```python
from build123d import *

# Parameters (mm, degrees)
TABAN_FLAN_1_DEPTH    = 10
IZIM2_R               = 25
IZIM2_R_2             = 4.25
IZIM2_R_3             = 5.5
IZIM2_R_4             = 3.25
KES_EKSTR_ZYON1_DEPTH = 10
RADYUS2_R             = 50
RADYUS3_R             = 30
RADYUS4_R             = 10
RADYUS5_R             = 50
RADYUS6_R             = 10
RADYUS7_R             = 5
IZIM3_R               = 2.5
KES_EKSTR_ZYON2_DEPTH = 29


# Sheet-metal steps are written as plain solids
with BuildPart() as part:
    # Çizim1 → Taban-Flanş1 (new body)
    with BuildSketch(Plane.XY):
        Polygon((0, 120), (-400, 120), (-400, 20), (-420, 20), (-420, -55), (-360, -55), (-330, -40), (-250, -40), (-200, -30), (-135, -30), (-135, -90), (-100, -90), (-100, -30), (0, -30), (0, 0), align=None)
    extrude(amount=-TABAN_FLAN_1_DEPTH)

    # Çizim2 → Kes-Ekstrüzyon1 (cut)
    with BuildSketch(Plane.XY):
        with Locations((-310, 45)):
            Circle(IZIM2_R)
        with Locations((-351.5, 86.5)):
            Circle(IZIM2_R_2)
        with Locations((-268.5, 86.5)):
            Circle(IZIM2_R_2)
        with Locations((-351.5, 3.5)):
            Circle(IZIM2_R_2)
        with Locations((-268.5, 3.5)):
            Circle(IZIM2_R_2)
        with Locations((-60, 55)):
            Circle(IZIM2_R_3)
        with Locations((-160, 55)):
            Circle(IZIM2_R_3)
        with Locations((-160, 15)):
            Circle(IZIM2_R_3)
        with Locations((-60, 15)):
            Circle(IZIM2_R_3)
        with Locations((-117.5, -75)):
            Circle(IZIM2_R_3)
        with Locations((-405, 10)):
            Circle(IZIM2_R_4)
        with Locations((-405, -40)):
            Circle(IZIM2_R_4)
    extrude(amount=-KES_EKSTR_ZYON1_DEPTH, mode=Mode.SUBTRACT)

    # Radyus2
    radyus2_edges = [part.edges().sort_by_distance(p)[0] for p in [
        (-400, 120, -5),
    ]]
    fillet(radyus2_edges, radius=RADYUS2_R)

    # Radyus3
    radyus3_edges = [part.edges().sort_by_distance(p)[0] for p in [
        (0, 120, -5),
    ]]
    fillet(radyus3_edges, radius=RADYUS3_R)

    # Radyus4
    radyus4_edges = [part.edges().sort_by_distance(p)[0] for p in [
        (0, -30, -5),
        (-100, -30, -5),
        (-100, -90, -5),
        (-135, -90, -5),
        (-135, -30, -5),
    ]]
    fillet(radyus4_edges, radius=RADYUS4_R)

    # Radyus5
    radyus5_edges = [part.edges().sort_by_distance(p)[0] for p in [
        (-200, -30, -5),
        (-250, -40, -5),
        (-330, -40, -5),
        (-360, -55, -5),
    ]]
    fillet(radyus5_edges, radius=RADYUS5_R)

    # Radyus6
    radyus6_edges = [part.edges().sort_by_distance(p)[0] for p in [
        (-420, -55, -5),
        (-420, 20, -5),
    ]]
    fillet(radyus6_edges, radius=RADYUS6_R)

    # Radyus7
    radyus7_edges = [part.edges().sort_by_distance(p)[0] for p in [
        (-400, 20, -5),
    ]]
    fillet(radyus7_edges, radius=RADYUS7_R)

    # Çizim3 → Kes-Ekstrüzyon2 (cut)
    with BuildSketch(Plane(origin=(0, 0, -10), x_dir=(-1, 0, 0), z_dir=(0, 0, -1))):
        with Locations((232.5, 72.5)):
            Circle(IZIM3_R)
        with Locations((232.5, 17.5)):
            Circle(IZIM3_R)
        with Locations((387.5, 17.5)):
            Circle(IZIM3_R)
        with Locations((387.5, 72.5)):
            Circle(IZIM3_R)
    extrude(amount=-KES_EKSTR_ZYON2_DEPTH, mode=Mode.SUBTRACT)


solid = part.part
```
Model file for the job. Use its own axes, mm. A direction names the side the tool comes from. Coordinates: 2 decimals unless noted, no trailing zeros. Order: outer loops, then holes, each group sorted by start corner. A loop starts at its lowest first (then second) coordinate and runs counter-clockwise, first axis right, second up. Notation, with made-up numbers: (-0.75, 14) - (46.25, 14) arc R18 cw to (46.25, 23) - close; hole circle Ø7 at (-19, 20.5). An arc over 180 degrees is marked (long way). Return JSON: item names as keys, results as strings. Group by question number.
1) Mould opens along Y. For faces 1 (the flat face through (-213, 40, -10)), 2 (the cylindrical face through (-65.495, 15.242, -4.93)), 3 (the flat face through (-345.06, -47.53, -4.93)) say: released by +Y, released by -Y, zero draft, split by the parting line, or undercut.
2) Tool access for faces 4 (the cylindrical face through (-360.47, -53.7, -5.07)), 5 (the flat face through (-51, -30, -5)), 6 (the cylindrical face through (-65.495, 55.242, -4.93)), 7 (the flat face through (-400, 48, -5)), 8 (the flat face through (-391, -55, -5)): list every direction of +Z, -Z, +X, -X, +Y, -Y with a clear straight run to the whole face (end or side of a thin tool).
3) Saw through at B-B, the plane y = -75. Write the cut outline in (x, z).
4) Saw through at A-A, the plane x = -60. Write the cut outline in (y, z), plus the area to 3 significant figures.
5) Flat gauge pins, fed straight in: P1, Ø9, axis at x = -117.5, y = -75, coming from the +Z side; P2, Ø1.5, axis at x = -351, z = -6, coming from the -Y side; P3, Ø1.5, axis at x = -74, z = -7, coming from the -Y side; P4, Ø1.5, axis at y = 60.5, z = -5.5, coming from the -X side. Where does each tip first touch, or does it go through?
6) Saw through at C-C, the plane x = -117.5. Write the cut outline in (y, z).
7) Probe line 1 (Y direction, x = -310, z = -6.5); line 2 (Y direction, x = -405, z = -3.5); line 3 (X direction, y = -76, z = -7.5). List the from-to ranges inside material, lowest first. Write a range as from..to.
8) Saw through at D-D, the plane y = 55. Write the cut outline in (x, z).
Values found:
{
 "1": {"face 1": "zero draft", "face 2": "undercut", "face 3": "released by -Y"},
 "2": {"face 4": "+Z, -Z, -Y", "face 5": "+Z, -Z, +X, -Y", "face 6": "+Z, -Z", "face 7": "+Z, -Z, -X, +Y", "face 8": "+Z, -Z, -X, -Y"},
 "3": {"outline": "(-135, -10) - (-123, -10) - (-123, 0) - (-135, 0) - close; (-112, -10) - (-100, -10) - (-100, 0) - (-112, 0) - close"},
 "4": {"outline": "(-30, -10) - (9.5, -10) - (9.5, 0) - (-30, 0) - close; (20.5, -10) - (49.5, -10) - (49.5, 0) - (20.5, 0) - close; (60.5, -10) - (120, -10) - (120, 0) - (60.5, 0) - close", "area": "1,280 mm²"},
 "5": {"P1": "passes through", "P2": "stops at y = -50.8", "P3": "stops at y = -30", "P4": "stops at x = -400"},
 "6": {"outline": "(-90, -10) - (-80.5, -10) - (-80.5, 0) - (-90, 0) - close; (-69.5, -10) - (120, -10) - (120, 0) - (-69.5, 0) - close"},
 "7": {"line 1": "y = -40..20, 70..120", "line 2": "y = -55..-43.25, -36.75..6.75, 13.25..20", "line 3": "x = -135..-122.91, -112.09..-100"},
 "8": {"outline": "(-400, -10) - (-332.91, -10) - (-332.91, 0) - (-400, 0) - close; (-287.09, -10) - (-165.5, -10) - (-165.5, 0) - (-287.09, 0) - close; (-154.5, -10) - (-65.5, -10) - (-65.5, 0) - (-154.5, 0) - close; (-54.5, -10) - (0, -10) - (0, 0) - (-54.5, 0) - close"}
}
